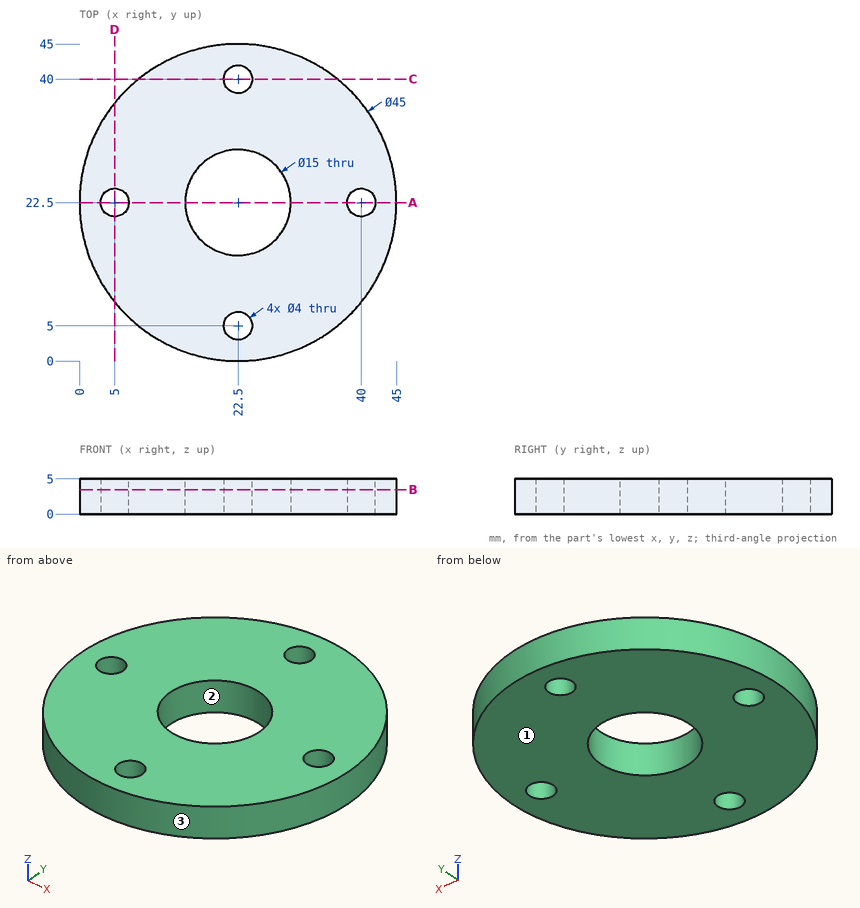
Here's the drawing with two shaded views (mm, measured from the low corner). I have some questions. Coordinates: 2 decimals unless noted, no trailing zeros. Loops run counter-clockwise (first coordinate to the right, second up) from the corner with the lowest first, then second, coordinate; pieces in that order, holes last. Notation, with made-up numbers: (18.25, 62) -> (62.25, 62) arc R27 ccw to (62.25, 90) -> close; hole circle Ø2 at (84, -31). An arc over 180 degrees is marked (long way). Use one line per item in the form item = value. Start each with the question number.
(1) If we section it at A-A (y = 22.5): Please give me the cut outline in (x, z).
(2) Please list where these lines run through material, in increasing order: line 1 along Y through (x, z) = (22.5, 3.3); line 2 along Y through (x, z) = (25, 0.6); line 3 along Y through (x, z) = (39.5, 3.3).
(3) If we section it at C-C (y = 40): Please give me the cut outline in (x, z), then the cut area to 3 significant figures.
(4) If we section it at B-B (z = 3.5): Please give me the cut outline in (x, y), then the cut area to 3 significant figures.
(5) Will this pin go through, and if not, where does the flat tip stop? pin 1 (2 mm diameter, centred on x = 20, z = 4, fed in from +Y).
(6) We'd pull the mould along X, two halves only. Please class the marked faces 1, 2 and 3: pulls with the +X half, pulls with the -X half, needs draft (parallel to the pull), parting line crosses it, or undercut.
Verdict:
q1.outline = (0, 0) -> (3, 0) -> (3, 5) -> (0, 5) -> close; (7, 0) -> (15, 0) -> (15, 5) -> (7, 5) -> close; (30, 0) -> (38, 0) -> (38, 5) -> (30, 5) -> close; (42, 0) -> (45, 0) -> (45, 5) -> (42, 5) -> close
q2.line_1 = 0 to 3, 7 to 15, 30 to 38, 42 to 45
q2.line_2 = 0.14 to 15.43, 29.57 to 44.86
q2.line_3 = 7.76 to 20.56, 24.44 to 37.24
q3.outline = (8.36, 0) -> (20.5, 0) -> (20.5, 5) -> (8.36, 5) -> close; (24.5, 0) -> (36.64, 0) -> (36.64, 5) -> (24.5, 5) -> close
q3.area = 121 mm²
q4.outline = circle Ø45 at (22.5, 22.5); hole circle Ø4 at (5, 22.5); hole circle Ø15 at (22.5, 22.5); hole circle Ø4 at (22.5, 5); hole circle Ø4 at (22.5, 40); hole circle Ø4 at (40, 22.5)
q4.area = 1,360 mm²
q5.pin_1 = 44.95
q6.face_1 = needs draft
q6.face_2 = undercut
q6.face_3 = parting line crosses it
